Study the drawing (mm; zero at the part's minimum x, y, z) and answer. Round coordinates to 2 decimals unless told otherwise and drop trailing zeros. Order: outer loops, then holes, each group sorted by start corner. A loop starts at its lowest first (then second) coordinate and runs counter-clockwise, first axis right, second up. Notation, with made-up numbers: M 48.25,-36.75 L 104.25,-36.75 A16 ccw 104.25,-16.75 Z; hole C -17,-16.75 d6. An arc over 180 degrees is marked long. Put each result on its own line as item: value. Start each with the question number.
1. The part is cut by section A-A (z = 6). Give the vertices of the cut face in (x, y), then the cut area to 3 significant figures.
2. The part is cut by section B-B (x = 12). Give the vertices of the cut face in (y, z), then the cut area to 3 significant figures.
3. The part is cut by section C-C (y = 0.85). Give the vertices of the cut face in (x, z).
4. Consider line 1 (Z direction, x = 29, y = 1.75); line 2 (X direction, y = 1, z = 40). Determine where each line is inside the solid, lowest interval first.
5. The mould has two halves that part along Z. Classify the marked faces 1, 2 and 3: +Z half, -Z half, draft (parallel to the pull), parting line (faces both ways), or undercut.
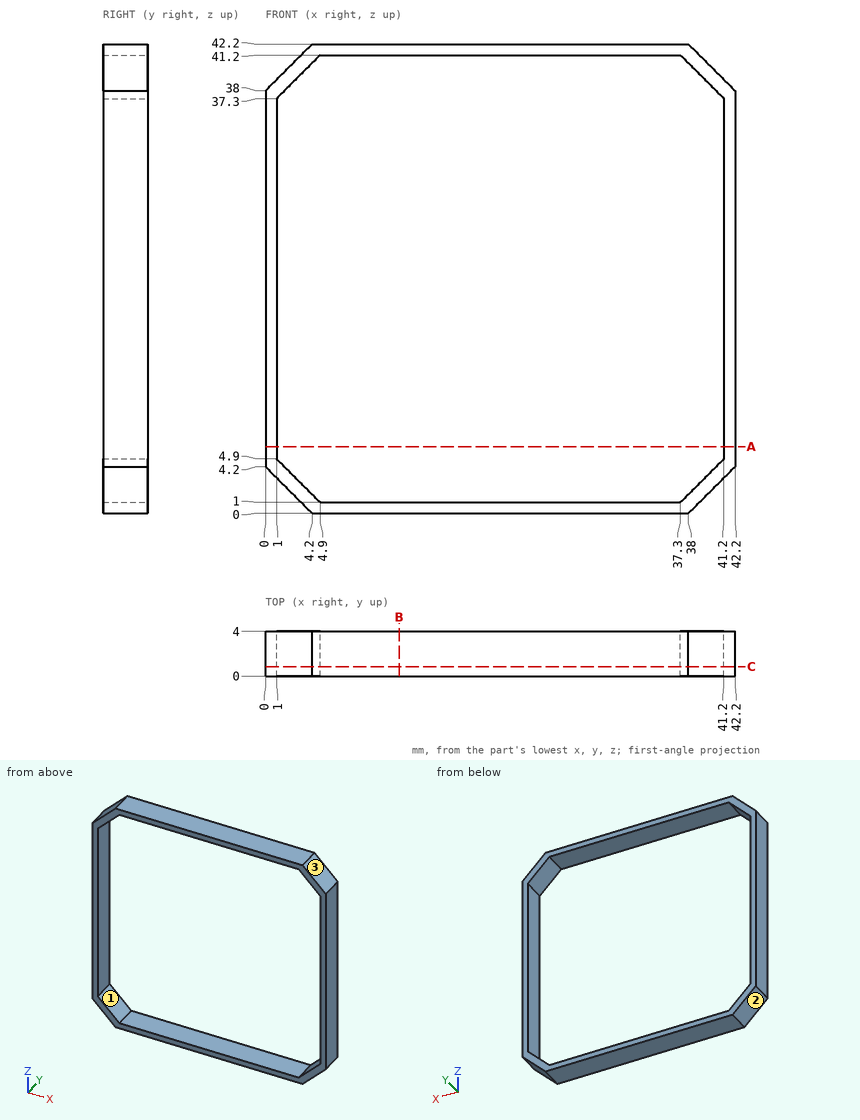
Resolved:
1. outline: M 0,0 L 1,0 L 1,4 L 0,4 Z; M 41.2,0 L 42.2,0 L 42.2,4 L 41.2,4 Z
1. area: 8.00 mm2
2. outline: M 0,0 L 4,0 L 4,1 L 0,1 Z; M 0,41.2 L 4,41.2 L 4,42.2 L 0,42.2 Z
2. area: 8.00 mm2
3. outline: M 0,4.2 L 4.2,0 L 38,0 L 42.2,4.2 L 42.2,38 L 38,42.2 L 4.2,42.2 L 0,38 Z; hole M 1,4.9 L 4.9,1 L 37.3,1 L 41.2,4.9 L 41.2,37.3 L 37.3,41.2 L 4.9,41.2 L 1,37.3 Z
4. line 1: 0 to 1, 41.2 to 42.2
4. line 2: 2 to 3.7, 38.5 to 40.2
5. face 1: undercut
5. face 2: -Z half
5. face 3: +Z half
